from build123d import *

# Parameters (mm, degrees)
M3_GEWINDEBOHRUNG1_D     = 2.5
M3_GEWINDEBOHRUNG1_DEPTH = 20
M3_GEWINDEBOHRUNG1_TIP   = 0.751075774


with BuildPart() as part:
    # Esboço1 → Revolução1 (revolve)
    with BuildSketch(Plane.XY, mode=Mode.PRIVATE) as revolu_o1_sk:
        Polygon((0, 0), (0, 40), (10, 40), (10, 35), (7.5, 34.5), (7.5, 33.5), (10, 33), (10, 26.5), (7.5, 25.75), (7.5, 24.25), (10, 23.5), (10, 15), (5, 10), (5, 0), align=None)
    revolve(revolu_o1_sk.sketch.rotate(Axis((0, 0, 0), (0, 1, 0)), 90), axis=Axis((0, 0, 0), (0, 1, 0)))

    # M3 Gewindebohrung1
    with Locations(Plane(origin=(0, 0, 0), x_dir=(0, 0, -1), z_dir=(0, -1, 0))):
        with Locations((0, 0)):
            Hole(M3_GEWINDEBOHRUNG1_D / 2, depth=M3_GEWINDEBOHRUNG1_DEPTH)
            with Locations((0, 0, -(M3_GEWINDEBOHRUNG1_DEPTH + M3_GEWINDEBOHRUNG1_TIP / 2))):  # 118° drill point
                Cone(0, M3_GEWINDEBOHRUNG1_D / 2, M3_GEWINDEBOHRUNG1_TIP, mode=Mode.SUBTRACT)


solid = part.part
Check sheet for the modelled part. Datum: model origin and axes. Units: mm. A direction names the side the tool comes from. Give positions to 0.01 mm unless a question says otherwise; leave off trailing zeros. Loops run counter-clockwise (first coordinate to the right, second up) from the corner with the lowest first, then second, coordinate; pieces in that order, holes last. Notation, with made-up numbers: M 80.5,81 L 95.5,81 A18 cw 95.5,86 Z; hole C -8,-4.5 d11. An arc over 180 degrees is marked long. Answer as a JSON object with one key per item and string values. Group by question number.
Q1. Material ranges on line 1 along Y through (x, z) = (-8, 2.75); line 2 along X through (y, z) = (5.5, 0); line 3 along Y through (x, z) = (6, -7.5), recorded low to high. Write a range as [from, to].
Q2. Cross-section at A-A on y = 12.5. Record the cut outline in (x, z), then the cut area to 3 significant figures.
Q3. Release check for a two-part mould opening along Z. For faces 4 (the cylindrical face through (-6.324, 24.99, -4.032)), 5 (the conical face through (-0.21, 20.62, 0.05)), 6 (the flat face through (0, 40, 0)) record: released by +Z, released by -Z, zero draft, split by the parting line, or undercut.
Q4. Access from +Z, -Z, +X, -X, +Y, -Y to the whole of each face (thin tool, end or side, straight path). Record for faces 1 (the conical face through (-2.3, 33.47, -7.3)), 2 (the cylindrical face through (0, 37, 10)), 3 (the cylindrical face through (-1.22, 10.14, -0.27)).
Q5. Cross-section at B-B on z = -8. Give the number of separate pieces and of enclosed holes in the cut face, then the cut area to 3 significant figures.
Q6. Cross-section at C-C on y = 31.5. Record the cut outline in (x, z), then the cut area to 3 significant figures.
Q7. Go/stop test with flat-tipped pins: P1, Ø1, axis at x = 5.5, y = 31.5, coming from the -Z side; P2, Ø8, axis at x = -7.5, z = -7, coming from the -Y side; P3, Ø6, axis at y = 8.5, z = -5, coming from the +X side. Record where each tip stops, or that it passes through.
Evaluation:
{
 "1": {"line 1": "y = [13.46, 23.96], [26.04, 33.31], [34.69, 40]", "line 2": "x = [-5, -1.25], [1.25, 5]", "line 3": "y = [14.6, 23.62], [26.38, 33.08], [34.92, 40]"},
 "2": {"outline": "C 0,0 d15; hole C 0,0 d2.5", "area": "172 mm2"},
 "3": {"face 4": "split by the parting line", "face 5": "undercut", "face 6": "zero draft"},
 "4": {"face 1": "none", "face 2": "+Y, -Y", "face 3": "-Y"},
 "5": {"separate pieces": "3", "enclosed holes": "0", "area": "271 mm2"},
 "6": {"outline": "C 0,0 d20", "area": "314 mm2"},
 "7": {"P1": "stops at z = -8.66", "P2": "stops at y = 11.26", "P3": "stops at x = 4.99"}
}
